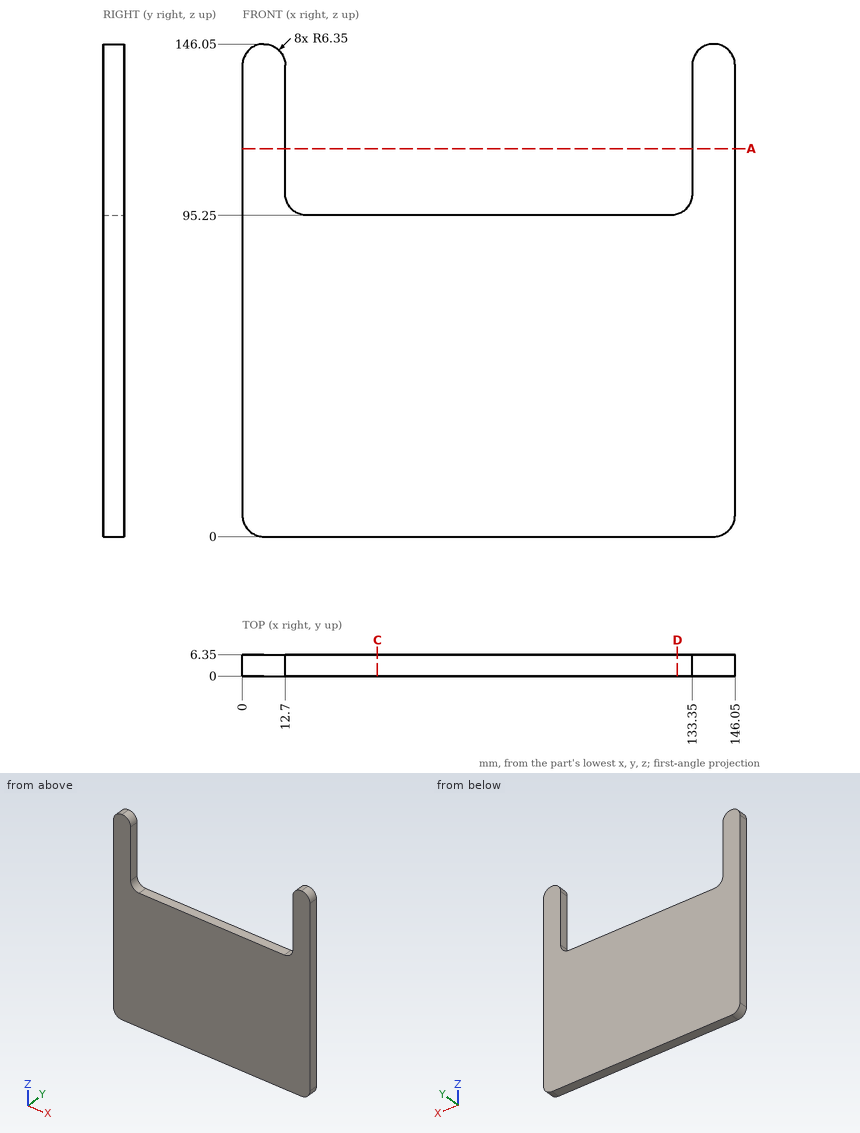
Source: three-view drawing plus pictorial views. Frame: mm from the lowest corner of the part. Give positions to 0.01 mm unless a question says otherwise; leave off trailing zeros. Loops run counter-clockwise (first coordinate to the right, second up) from the corner with the lowest first, then second, coordinate; pieces in that order, holes last. Notation, with made-up numbers: (54, 47) -> (106, 47) arc R17 cw to (106, 68) -> close; hole circle Ø3 at (-36.75, 58.5). An arc over 180 degrees is marked (long way). Put each result on its own line as item: value. Start each with the question number.
1) Cut plane C-C (x = 40). Return loops of the section in (y, z).
2) Material intervals for probe 1 along X at (y, z) = (2, 129.5); probe 2 along Z at (x, y) = (71, 1.25); probe 3 along X at (y, z) = (2, 96), sorted ascending.
3) Contact query for flat-ended pins moving along their axis: P1, Ø1.5, axis at x = 119, y = 5.5, coming from the +Z side; P2, Ø1.5, axis at x = 117, y = 2.5, coming from the -Z side; P3, Ø3, axis at x = 17, y = 3, coming from the +Z side (3 decimals). Output: stop coordinate, or through.
4) Cut plane A-A (z = 115). Return loops of the section in (x, y).
5) Cut plane D-D (x = 129). Return loops of the section in (y, z).
Results are:
1. outline: (0, 0) -> (6.35, 0) -> (6.35, 95.25) -> (0, 95.25) -> close
2. probe 1: x = 0 to 12.7, 133.35 to 146.05
2. probe 2: z = 0 to 95.25
2. probe 3: x = 0 to 16.06, 129.99 to 146.05
3. P1: stops at z = 95.25
3. P2: stops at z = 0
3. P3: stops at z = 96.335
4. outline: (0, 0) -> (12.7, 0) -> (12.7, 6.35) -> (0, 6.35) -> close; (133.35, 0) -> (146.05, 0) -> (146.05, 6.35) -> (133.35, 6.35) -> close
5. outline: (0, 0) -> (6.35, 0) -> (6.35, 95.57) -> (0, 95.57) -> close
